Model file for the job. Use its own axes, mm. A direction names the side the tool comes from. Give positions to 0.01 mm unless a question says otherwise; leave off trailing zeros. Write each loop counter-clockwise with the first axis right and the second up, starting at its lowest first coordinate (ties: lowest second). Pieces come first, ordered by that corner, then holes. Notation, with made-up numbers: (-32.5, 31.5) - (-22.5, 31.5) arc R22 cw to (-22.5, 55.5) - close; hole circle Ø9 at (-28.5, 71). An arc over 180 degrees is marked (long way). One line per item, written item: value. Start each with the question number.
(1) 3-axis set-ups, long thin cutter, end or side, ignore diameter. For faces 1 (the face through (-222.865, 42.519, 0.661)), 2 (the face through (-208, 249, 3)), 3 (the face through (-207, 46.463, -6)): which of +Z, -Z, +X, -X, +Y, -Y reach the whole face in a straight line?
(2) Cut at B-B, the plane z = -6.5. List the corners of the cut face in (x, y), and give its area (3 significant figures).
(3) Drop flat-ended pins along their axis: P1, Ø8, axis at y = 159.5, z = 8.5, coming from the -X side; P2, Ø15, axis at x = -210, y = 202.5, coming from the -Z side; P3, Ø4, axis at x = -204, z = 8, coming from the +Y side; P4, Ø11, axis at x = -210.5, z = -4.5, coming from the +Y side. Give the stop position or say it passes through.
(4) Mould opens along Y. For faces 4 (the face through (-204.35, 424.81, 1.52)), 5 (the face through (-208, 249, 0)), 6 (the face through (-209, 46.463, 9)), 7 (the face through (-208, 38.463, 2)) say: pulls with the +Y half, pulls with the -Y half, needs draft (parallel to the pull), parting line crosses it, or undercut.
(5) Cut at A-A, the plane y = 209. List the corners of the cut face in (x, z).
(6) Probe L1, parallel to Y at x = -210.5, z = -12; L2, parallel to Z at x = -219, y = 301; L3, parallel to Y at x = -204, z = 1. List the from-to ranges inside material, lowest first.
from build123d import *

# Parameters (mm, degrees)
SZKIC1_W                    = 30
SZKIC1_H                    = 400
DODANIE_WYCI_GNI_CIE1_DEPTH = 3
SZKIC2_R                    = 7.5
WYTNIJ_WYCI_GNI_CIE1_DEPTH  = 3
SZKIC3_R                    = 15.074813432
DODANIE_WYCI_GNI_CIE2_DEPTH = 8


with BuildPart() as part:
    # Szkic1 → Dodanie-wyciągnięcie1 (new body)
    with BuildSketch(Plane.XY):
        with Locations((-207.813580858, 246.462746709)):
            Rectangle(SZKIC1_W, SZKIC1_H)
    extrude(amount=DODANIE_WYCI_GNI_CIE1_DEPTH)

    # Szkic2 → Wytnij-wyciągnięcie1 (cut)
    with BuildSketch(Plane.XY.offset(3)):
        with Locations((-207.813580858, 431.462746709)):
            Circle(SZKIC2_R)
    extrude(amount=-WYTNIJ_WYCI_GNI_CIE1_DEPTH, mode=Mode.SUBTRACT)

    # Szkic3 → Dodanie-wyciągnięcie2 (add)
    with BuildSketch(Plane.XZ.offset(-46.462746709)):
        with Locations(Location((-207.813580858, 1.5, 0), (0, 0, 5.710593137))):
            Circle(SZKIC3_R)
    extrude(amount=DODANIE_WYCI_GNI_CIE2_DEPTH)


solid = part.part
Answers follow:
1. face 1: +Y, -Y
1. face 2: +Z, +X, -X, +Y
1. face 3: -Z, +X, -X, +Y
2. outline: (-220.59, 38.46) - (-195.04, 38.46) - (-195.04, 46.46) - (-220.59, 46.46) - close
2. area: 204 mm²
3. P1: passes through
3. P2: stops at z = 0
3. P3: stops at y = 46.46
3. P4: stops at y = 446.46
4. face 4: undercut
4. face 5: needs draft
4. face 6: pulls with the +Y half
4. face 7: pulls with the -Y half
5. outline: (-222.81, 0) - (-192.81, 0) - (-192.81, 3) - (-222.81, 3) - close
6. L1: y = 38.46 to 46.46
6. L2: z = 0 to 3
6. L3: y = 38.46 to 425, 437.92 to 446.46
